Source: CAD feature listing. Evaluate the final solid. Frame: model axes, mm. Face numbers are marked on the shaded views. Round coordinates to 2 decimals unless told otherwise and drop trailing zeros. Loops run counter-clockwise (first coordinate to the right, second up) from the corner with the lowest first, then second, coordinate; pieces in that order, holes last. Notation, with made-up numbers: M 36,31.5 L 82,31.5 A20 ccw 82,47.5 Z; hole C -28,-23.75 d7. An arc over 180 degrees is marked long. Write each question's results on one line, items separated by ' | '. Start each with the question number.
1. Draft query along Y for the marked faces 1 and 2. Return one class per face: released by +Y, released by -Y, zero draft, split by the parting line, or undercut.
2. Contact query for flat-ended pins moving along their axis: pin 1 Ø9 at (x, y) = (-80, 14) entering from +Z; pin 2 Ø6.5 at (x, y) = (45, 18.36) entering from +Z; pin 3 Ø3 at (x, z) = (-10.5, 1.5) entering from -Y; pin 4 Ø10 at (x, y) = (-50, 10.5) entering from -Z. Output: stop coordinate, or through.
3. Ray query, line 1 (Z direction, x = 13, y = 21); line 2 (Y direction, x = -80, z = 4.05); line 3 (Y direction, x = -17, z = 5.2). Return the intervals inside material, ascending.
4. Section A-A on z = 4.15. Output: boundary loops of the cut face in (x, y).
from build123d import *

# Parameters (mm, degrees)
F0_R     = 8.5
F0_R_2   = 8
F0_R_3   = 4
F0_R_4   = 7.5
F0_R_5   = 7
F0_R_6   = 6.5
F1_DEPTH = 6
F3_DEPTH = 3


# Not quite as in the source:
# - ends of sketch curves that miss each other by under 0.0002 mm in the source are joined


with BuildPart() as f1:
    # F0 (on Top) → F1 (new body)
    with BuildSketch(Plane.XY):
        with BuildLine():
            ThreePointArc((44.5540603798, 26.8468655378), (-17.2418869333, 25.5132571498), (-79.0021794007, 28))
            ThreePointArc((-79.0021794007, 28), (-94.0355137401, 14), (-79.0021794007, 0))
            ThreePointArc((-79.0021794007, 0), (-16.5001968513, 3.3088101205), (45.7422348275, 9.8910396618))
            ThreePointArc((45.7422348275, 9.8910396618), (53.4792070742, 18.9527489424), (44.5540603798, 26.8468655378))
        make_face()
        with Locations((-60.0031413922, 13.6455344589)):
            Circle(F0_R, mode=Mode.SUBTRACT)
        with Locations((-38.7143914059, 13.7077101978)):
            Circle(F0_R_2, mode=Mode.SUBTRACT)
        with Locations((-80, 14)):
            Circle(F0_R_3, mode=Mode.SUBTRACT)
        with Locations((-17.4317891816, 14.2230589801)):
            Circle(F0_R_4, mode=Mode.SUBTRACT)
        with Locations((3.8350196915, 15.191347242)):
            Circle(F0_R_5, mode=Mode.SUBTRACT)
        with Locations((25.0763967822, 16.6121361411)):
            Circle(F0_R_6, mode=Mode.SUBTRACT)
        with Locations((45, 18.3585710294)):
            Circle(F0_R_3, mode=Mode.SUBTRACT)
    extrude(amount=F1_DEPTH)

    # F2 (on Top) → F3 (cut)
    with BuildSketch(Plane.XY):
        with BuildLine():
            Line((48.3999060802, 23.8845237164), (-85.0995088492, 23.4892851738))
            ThreePointArc((-85.0995088492, 23.4892851738), (-86.3603062967, 13.0242161587), (-85.7702605867, 2.5))
            Line((-85.7702605867, 2.5), (48.4354331402, 11.884576307))
            ThreePointArc((48.4354331402, 11.884576307), (49.0927734894, 17.8865487251), (48.3999060802, 23.8845237164))
        make_face()
    extrude(amount=F3_DEPTH, mode=Mode.SUBTRACT)


solid = f1.part
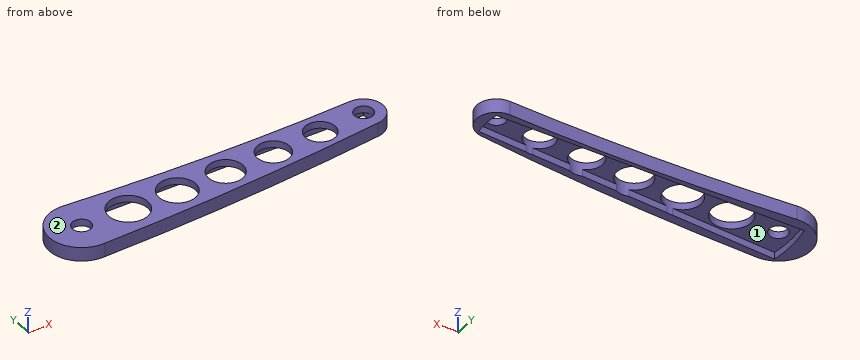
Taken from the geometry:
1) face 1: undercut | face 2: zero draft
2) pin 1: z = 6 | pin 2: through | pin 3: y = 3.67 | pin 4: z = 3
3) line 1: 3 to 6 | line 2: -0.04 to 10, 18 to 28.04 | line 3: 3.27 to 6.74, 21.71 to 25.51
4) outline: M -79,0 A1193 ccw 45.74,9.89 A8.5 ccw 44.55,26.85 A1000 cw -79,28 A14.04 ccw long Z; hole C -80,14 d8; hole C -60,13.65 d17; hole C -38.71,13.71 d16; hole C -17.43,14.22 d15; hole C 3.84,15.19 d14; hole C 25.08,16.61 d13; hole C 45,18.36 d8
